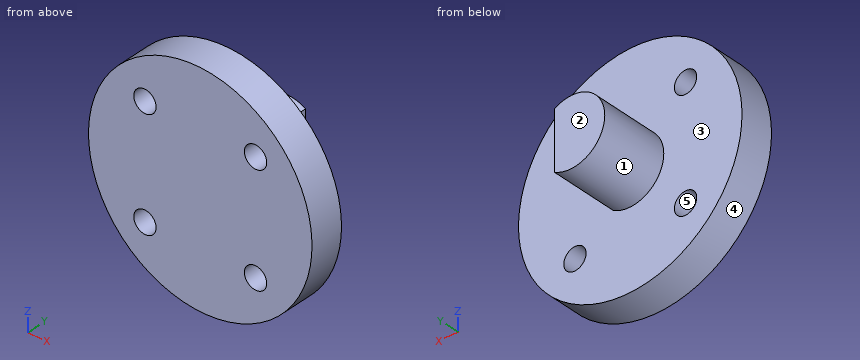
from build123d import *

# Parameters (mm, degrees)
CROQUIS1_R              = 10
CROQUIS1_R_2            = 1
SALIENTE_EXTRUIR1_DEPTH = 3
SALIENTE_EXTRUIR2_START = 3
CROQUIS1_3_R            = 3
SALIENTE_EXTRUIR2_DEPTH = 6
CORTAR_EXTRUIR1_START   = -6
CORTAR_EXTRUIR1_DEPTH   = 6


with BuildPart() as part:
    # Croquis1 → Saliente-Extruir1 (new body)
    with BuildSketch(Plane(origin=(0, 0, 0), x_dir=(1, 0, 0), z_dir=(0, 1, 0))):
        with Locations(Location((0, 0, 0), (0, 0, 270))):
            Circle(CROQUIS1_R)
        with Locations(Location((-4.949747468, 4.949747468, 0), (0, 0, 270))):
            Circle(CROQUIS1_R_2, mode=Mode.SUBTRACT)
        with Locations(Location((4.949747468, 4.949747468, 0), (0, 0, 270))):
            Circle(CROQUIS1_R_2, mode=Mode.SUBTRACT)
        with Locations(Location((4.949747468, -4.949747468, 0), (0, 0, 270))):
            Circle(CROQUIS1_R_2, mode=Mode.SUBTRACT)
        with Locations(Location((-4.949747468, -4.949747468, 0), (0, 0, 270))):
            Circle(CROQUIS1_R_2, mode=Mode.SUBTRACT)
    extrude(amount=SALIENTE_EXTRUIR1_DEPTH)

    # Croquis1<3> → Saliente-Extruir2 (add)
    with BuildSketch(Plane(origin=(0, 0, 0), x_dir=(1, 0, 0), z_dir=(0, 1, 0)).offset(SALIENTE_EXTRUIR2_START)):
        with Locations(Location((0, 0, 0), (0, 0, 270))):
            Circle(CROQUIS1_3_R)
    extrude(amount=SALIENTE_EXTRUIR2_DEPTH)

    # Croquis2 → Cortar-Extruir1 (cut)
    with BuildSketch(Plane(origin=(0, 9, 0), x_dir=(1, 0, 0), z_dir=(0, 1, 0)).offset(CORTAR_EXTRUIR1_START)):
        with BuildLine():
            Line((1.5, 2.598076211), (1.5, -2.598076211))
            ThreePointArc((1.5, -2.598076211), (3, 0), (1.5, 2.598076211))
        make_face()
    extrude(amount=CORTAR_EXTRUIR1_DEPTH, mode=Mode.SUBTRACT)


solid = part.part
Check sheet for the modelled part. Datum: model origin and axes. Units: mm. Face numbers are marked on the shaded views. A direction names the side the tool comes from. Round coordinates to 2 decimals unless told otherwise and drop trailing zeros. Order: outer loops, then holes, each group sorted by start corner. A loop starts at its lowest first (then second) coordinate and runs counter-clockwise, first axis right, second up.
Q1. Cross-section at C-C, the plane x = 5.5. Enter the section's corners in (y, z).
Filled sheet:
outline: (0, -8.35) - (3, -8.35) - (3, -5.78) - (0, -5.78) - close; (0, -4.11) - (3, -4.11) - (3, 4.11) - (0, 4.11) - close; (0, 5.78) - (3, 5.78) - (3, 8.35) - (0, 8.35) - close
Q2. Scan lines: L1, parallel to X at y = 1, z = -5; L2, parallel to X at y = 2.5, z = -5.25; L3, parallel to Y at x = 1, z = 6.25. Record each from-to range of solid material in increasing order.
Filled sheet:
L1: x = -8.66 to -5.95, -3.95 to 3.95, 5.95 to 8.66
L2: x = -8.51 to -5.9, -4 to 4, 5.9 to 8.51
L3: y = 0 to 3
Q3. Set-up check for the marked faces 1 and 2: record each of +Z, -Z, +X, -X, +Y, -Y from which the full face is reachable in a straight line by a thin tool's end or side.
Filled sheet:
face 1: +Y
face 2: +Z, -Z, +X, -X, +Y
Q4. Draft check along Z on the marked faces 3, 4 and 5. Enter one of: pulls with the +Z half, pulls with the -Z half, needs draft (parallel to the pull), parting line crosses it, or undercut.
Filled sheet:
face 3: needs draft
face 4: parting line crosses it
face 5: undercut
Q5. Cross-section at A-A, the plane x = 0. Enter the section's corners in (y, z).
Filled sheet:
outline: (0, -10) - (3, -10) - (3, -3) - (9, -3) - (9, 3) - (3, 3) - (3, 10) - (0, 10) - close
Q6. Depth check by flat-ended pin: P1, Ø3, axis at x = 4.95, z = -4.95, coming from the +Y side; P2, Ø1.6, axis at y = 5, z = -0.5, coming from the +X side. Enter the tip coordinate at first touch or a pass-through.
Filled sheet:
P1: stops at y = 3
P2: stops at x = 1.5
Q7. Cross-section at B-B, the plane z = 0. Enter the section's corners in (x, y).
Filled sheet:
outline: (-10, 0) - (10, 0) - (10, 3) - (1.5, 3) - (1.5, 9) - (-3, 9) - (-3, 3) - (-10, 3) - close
Q8. Cross-section at D-D, the plane y = 5.75. Enter the section's corners in (x, z).
Filled sheet:
outline: (1.5, -2.6) - (1.5, 2.6) arc R3 ccw (long way) to start
